The model under review builds one solid part; all positions refer to its coordinate system, in mm. Face numbers are marked on the shaded views. A direction names the side the tool comes from. Coordinates: 2 decimals unless noted, no trailing zeros. Write each loop counter-clockwise with the first axis right and the second up, starting at its lowest first coordinate (ties: lowest second). Pieces come first, ordered by that corner, then holes. Notation, with made-up numbers: (-7, 39) - (35, 39) arc R32 ccw to (35, 76) - close; hole circle Ø9 at (65, 83). An arc over 180 degrees is marked (long way). Return JSON: item names as keys, results as strings. Group by question number.
(1) We need section C-C on x = 6.75. State the section outline as (y, z) points.
(2) We need section D-D on y = 20.75. State the section outline as (x, z) points.
(3) To check wall thickness, follow L1, parallel to X at y = 41.5, z = 48.5; L2, parallel to X at y = 41.5, z = 45.5; L3, parallel to Y at x = 4.25, z = 44.75. State the ranges of each line that lie inside material, in increasing order. Write a range as from..to.
(4) For pin 1 Ø3 at (x, y) = (2, 32.5) entering from -Z; pin 2 Ø2 at (y, z) = (30.5, 39) entering from +X; pin 3 Ø3.5 at (x, y) = (-4.5, 18) entering from +Z; pin 4 Ø5 at (x, y) = (-6.5, 24.5) entering from -Z, all flat-tipped, find the tip position at first contact; note any pin that passes through.
(5) Tool access review of the marked faces 1, 2, 3, 4 and 5: name each direction out of +Z, -Z, +X, -X, +Y, -Y from which nothing blocks a thin tool from reaching the whole face with its end or side.
```python
from build123d import *

# Parameters (mm, degrees)
SKETCH014_W  = 20
SKETCH014_H  = 10
SKETCH014_R  = 1.5
PAD006_DEPTH = 3
SKETCH015_W  = 10
SKETCH015_H  = 10
PAD007_DEPTH = 12
SKETCH028_W  = 10
SKETCH028_H  = 20
PAD014_DEPTH = 3
PAD015_DEPTH = 10
SKETCH029_W  = 5.341147
SKETCH029_H  = 20
PAD016_DEPTH = 10
PAD017_DEPTH = 10
FILLET001_R  = 1
FILLET002_R  = 1
FILLET003_R  = 1


with BuildPart() as part:
    # Sketch014 → Pad006 (new body)
    with BuildSketch(Plane(origin=(0, 16.63325, 0), x_dir=(-1, 0, 0), z_dir=(0, 1, 0))):
        with Locations((0.000853, 44.999577)):
            Rectangle(SKETCH014_W, SKETCH014_H)
        with Locations((-6.55861, 47.39436)):
            Circle(SKETCH014_R, mode=Mode.SUBTRACT)
        with Locations((-6.556974, 42.39436)):
            Circle(SKETCH014_R, mode=Mode.SUBTRACT)
    extrude(amount=PAD006_DEPTH)

    # Sketch015 (on Face8 of Pad006) → Pad007 (join)
    with BuildSketch(Plane(origin=(-10, 19.63325, 0), x_dir=(-1, 0, 0), z_dir=(0, 1, 0))):
        with Locations((-5, 44.980343)):
            Rectangle(SKETCH015_W, SKETCH015_H)
    extrude(amount=PAD007_DEPTH)

    # Sketch028 → Pad014 (join)
    with BuildSketch(Plane(origin=(0, 31.63, 0), x_dir=(-1, 0, 0), z_dir=(0, 1, 0))):
        with Locations((5.002885, 45.155186)):
            Rectangle(SKETCH028_W, SKETCH028_H)
    extrude(amount=PAD014_DEPTH)

    # Sketch027 → Pad015 (join)
    with BuildSketch(Plane(origin=(-2, 34.63, 45), x_dir=(1, 0, 0), z_dir=(0, 1, 0))):
        with BuildLine():
            Line((1.975717, 9.843815), (-0.708844, 9.843815))
            Line((-1.566561, 9.843815), (-0.708844, 9.843815))
            ThreePointArc((-1.566561, 9.843815), (-1.674924, 9.798929), (-1.71981, 9.690566))
            Line((-1.71981, 8.956594), (-1.71981, 9.690566))
            ThreePointArc((-1.71981, 8.956594), (-1.675937, 8.850677), (-1.57002, 8.806804))
            Line((-0.809443, 8.806804), (-1.57002, 8.806804))
            ThreePointArc((-0.704389, 8.701751), (-0.735158, 8.776035), (-0.809443, 8.806804))
            Line((-0.704389, 8.026948), (-0.704389, 8.701751))
            ThreePointArc((-0.916234, 7.815103), (-0.766437, 7.877151), (-0.704389, 8.026948))
            Line((-1.56111, 7.815103), (-0.916234, 7.815103))
            ThreePointArc((-1.56111, 7.815103), (-1.661811, 7.773391), (-1.703522, 7.672691))
            Line((-1.703522, 6.956427), (-1.703522, 7.672691))
            ThreePointArc((-1.703522, 6.956427), (-1.662049, 6.856302), (-1.561925, 6.81483))
            Line((-0.810564, 6.81483), (-1.561925, 6.81483))
            ThreePointArc((-0.703462, 6.707728), (-0.734831, 6.78346), (-0.810564, 6.81483))
            Line((-0.703462, 6.007832), (-0.703462, 6.707728))
            ThreePointArc((-0.892518, 5.818776), (-0.758835, 5.874149), (-0.703462, 6.007832))
            Line((-1.561271, 5.818776), (-0.892518, 5.818776))
            ThreePointArc((-1.561271, 5.818776), (-1.661881, 5.777102), (-1.703555, 5.676492))
            Line((-1.703555, 4.96034), (-1.703555, 5.676492))
            ThreePointArc((-1.703555, 4.96034), (-1.662091, 4.860238), (-1.56199, 4.818775))
            Line((-0.810665, 4.818775), (-1.56199, 4.818775))
            ThreePointArc((-0.703555, 4.711665), (-0.734926, 4.787403), (-0.810665, 4.818775))
            Line((-0.703555, 4.022301), (-0.703555, 4.711665))
            ThreePointArc((-0.903152, 3.822704), (-0.762015, 3.881164), (-0.703555, 4.022301))
            Line((-1.561369, 3.822704), (-0.903152, 3.822704))
            ThreePointArc((-1.561369, 3.822704), (-1.661978, 3.78103), (-1.703652, 3.680421))
            Line((-1.703652, 2.964269), (-1.703652, 3.680421))
            ThreePointArc((-1.703652, 2.964269), (-1.662188, 2.864167), (-1.562087, 2.822704))
            Line((-0.810762, 2.822704), (-1.562087, 2.822704))
            ThreePointArc((-0.703652, 2.715594), (-0.735023, 2.791332), (-0.810762, 2.822704))
            Line((-0.703652, 2.011374), (-0.703652, 2.715594))
            ThreePointArc((-0.888393, 1.826633), (-0.757761, 1.880742), (-0.703652, 2.011374))
            Line((-1.561466, 1.826633), (-0.888393, 1.826633))
            ThreePointArc((-1.561466, 1.826633), (-1.662075, 1.784959), (-1.703749, 1.68435))
            Line((-1.703749, 0.968198), (-1.703749, 1.68435))
            ThreePointArc((-1.703749, 0.968198), (-1.662285, 0.868096), (-1.562184, 0.826633))
            Line((-0.810859, 0.826633), (-1.562184, 0.826633))
            ThreePointArc((-0.703749, 0.719523), (-0.73512, 0.795261), (-0.810859, 0.826633))
            Line((-0.703749, 0.000302), (-0.703749, 0.719523))
            ThreePointArc((-0.873489, -0.169438), (-0.753464, -0.119723), (-0.703749, 0.000302))
            Line((-1.561563, -0.169438), (-0.873489, -0.169438))
            ThreePointArc((-1.561563, -0.169438), (-1.662172, -0.211112), (-1.703846, -0.311721))
            Line((-1.703846, -1.027873), (-1.703846, -0.311721))
            ThreePointArc((-1.703846, -1.027873), (-1.662382, -1.127975), (-1.562281, -1.169438))
            Line((-0.810956, -1.169438), (-1.562281, -1.169438))
            ThreePointArc((-0.703846, -1.276548), (-0.735217, -1.20081), (-0.810956, -1.169438))
            Line((-0.703846, -1.973203), (-0.703846, -1.276548))
            ThreePointArc((-0.896152, -2.165509), (-0.760171, -2.109184), (-0.703846, -1.973203))
            Line((-1.56166, -2.165509), (-0.896152, -2.165509))
            ThreePointArc((-1.56166, -2.165509), (-1.662269, -2.207183), (-1.703943, -2.307792))
            Line((-1.703943, -3.023944), (-1.703943, -2.307792))
            ThreePointArc((-1.703943, -3.023944), (-1.662479, -3.124046), (-1.562378, -3.165509))
            Line((-0.811053, -3.165509), (-1.562378, -3.165509))
            ThreePointArc((-0.703943, -3.272619), (-0.735314, -3.196881), (-0.811053, -3.165509))
            Line((-0.703943, -3.990733), (-0.703943, -3.272619))
            ThreePointArc((-0.87479, -4.16158), (-0.753983, -4.11154), (-0.703943, -3.990733))
            Line((-1.561757, -4.16158), (-0.87479, -4.16158))
            ThreePointArc((-1.561757, -4.16158), (-1.662366, -4.203254), (-1.70404, -4.303863))
            Line((-1.70404, -5.020015), (-1.70404, -4.303863))
            ThreePointArc((-1.70404, -5.020015), (-1.662576, -5.120117), (-1.562475, -5.16158))
            Line((-0.81115, -5.16158), (-1.562475, -5.16158))
            ThreePointArc((-0.70404, -5.26869), (-0.735411, -5.192952), (-0.81115, -5.16158))
            Line((-0.70404, -5.994353), (-0.70404, -5.26869))
            ThreePointArc((-0.867338, -6.157651), (-0.751869, -6.109822), (-0.70404, -5.994353))
            Line((-1.561854, -6.157651), (-0.867338, -6.157651))
            ThreePointArc((-1.561854, -6.157651), (-1.662463, -6.199325), (-1.704137, -6.299934))
            Line((-1.704137, -7.016086), (-1.704137, -6.299934))
            ThreePointArc((-1.704137, -7.016086), (-1.662673, -7.116188), (-1.562572, -7.157651))
            Line((-0.811247, -7.157651), (-1.562572, -7.157651))
            ThreePointArc((-0.704137, -7.264761), (-0.735508, -7.189023), (-0.811247, -7.157651))
            Line((-0.704137, -8.006283), (-0.704137, -7.264761))
            ThreePointArc((-0.851576, -8.153722), (-0.747321, -8.110538), (-0.704137, -8.006283))
            Line((-1.561951, -8.153722), (-0.851576, -8.153722))
            ThreePointArc((-1.561951, -8.153722), (-1.671215, -8.198981), (-1.716474, -8.308246))
            Line((-1.716474, -8.999917), (-1.716474, -8.308246))
            ThreePointArc((-1.716474, -8.999917), (-1.671425, -9.108674), (-1.562669, -9.153722))
            Line((-0.811344, -9.153722), (-1.562669, -9.153722))
            ThreePointArc((-0.704234, -9.260832), (-0.735605, -9.185094), (-0.811344, -9.153722))
            Line((-0.704234, -10.153722), (-0.704234, -9.260832))
            Line((-0.704234, -10.153722), (1.975717, -10.153722))
            Line((1.975717, -10.153722), (1.975717, 9.843815))
        make_face()
    extrude(amount=PAD015_DEPTH)

    # Sketch029 → Pad016 (join)
    with BuildSketch(Plane(origin=(0, 34.63, 0), x_dir=(-1, 0, 0), z_dir=(0, 1, 0))):
        with Locations((7.333255, 45.149561)):
            Rectangle(SKETCH029_W, SKETCH029_H)
    extrude(amount=PAD016_DEPTH)

    # Sketch035 (on Face15 of Pad016) → AdditiveLoft002 section 0
    with BuildSketch(Plane(origin=(-0.002885, 16.63325, 0), x_dir=(0, 0, -1), z_dir=(1, 0, 0))):
        Polygon((-55.139091, 14.987795), (-49.973751, 14.987795), (-49.973751, 4.987795), align=None)
    # Sketch036 (on Face15 of Pad016) → AdditiveLoft002 section 1
    with BuildSketch(Plane(origin=(-10.002885, 16.63325, 0), x_dir=(0, 0, -1), z_dir=(1, 0, 0))):
        Polygon((-55.139091, 14.987795), (-49.973751, 14.987795), (-49.973751, 4.987795), align=None)
    loft()

    # Sketch037 (on Face19 of AdditiveLoft002) → Pad017 (join)
    with BuildSketch(Plane(origin=(-0.002885, 16.63325, 0), x_dir=(0, 0, -1), z_dir=(1, 0, 0))):
        Polygon((-39.968193, 15.033547), (-35.187713, 15.033547), (-39.968193, 5.033547), align=None)
    extrude(amount=-PAD017_DEPTH)

    # Fillet001
    fillet001_edges = [part.edges().sort_by_distance(p)[0] for p in [
        (9.999147, 19.63325, 44.999577),
    ]]
    fillet(fillet001_edges, radius=FILLET001_R)

    # Fillet002
    fillet002_edges = [part.edges().sort_by_distance(p)[0] for p in [
        (-0.024283, 44.63, 45.154954),
    ]]
    fillet(fillet002_edges, radius=FILLET002_R)

    # Fillet003
    fillet003_edges = [part.edges().sort_by_distance(p)[0] for p in [
        (-10.003829, 44.63, 45.149561),
    ]]
    fillet(fillet003_edges, radius=FILLET003_R)


solid = part.part
```
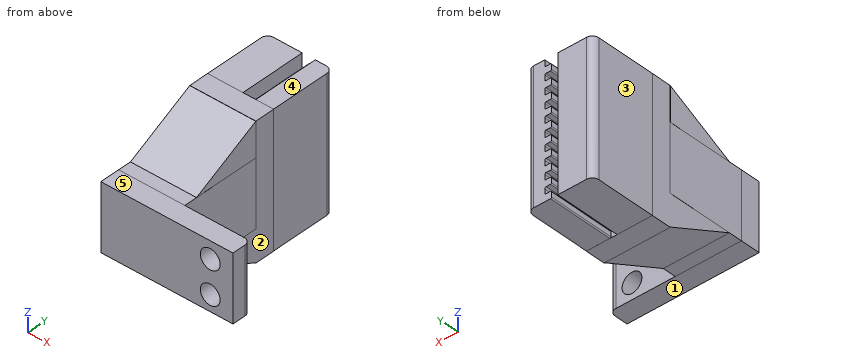
Ans:
{
 "1": {"outline": "(16.63, 40) - (19.63, 40) - (19.63, 40.91) - (16.63, 40.91) - close; (16.63, 43.88) - (19.63, 43.88) - (19.63, 45.91) - (16.63, 45.91) - close; (16.63, 48.88) - (19.63, 48.88) - (19.63, 50) - (16.63, 50) - close"},
 "2": {"outline": "(-10, 39.98) - (0, 39.98) - (0, 49.98) - (-10, 49.98) - close"},
 "3": {"L1": "-10..-4.66, -2.7..-0.02", "L2": "-10..-4.66, -3.7..-0.02", "L3": "16.63..19.63"},
 "4": {"pin 1": "through", "pin 2": "x = 0", "pin 3": "z = 50", "pin 4": "z = 37.42"},
 "5": {"face 1": "-Z, +X, -X, -Y", "face 2": "+Z, -Z, +X, +Y", "face 3": "+Z, -Z, -X, +Y, -Y", "face 4": "+Z, +X, -X, +Y, -Y", "face 5": "+Z, +X, -X, -Y"}
}
